Source: three-view drawing plus pictorial views. Frame: mm from the lowest corner of the part. Give positions to 0.01 mm unless a question says otherwise; leave off trailing zeros. Write each loop counter-clockwise with the first axis right and the second up, starting at its lowest first coordinate (ties: lowest second). Pieces come first, ordered by that corner, then holes. Notation, with made-up numbers: (86, -3) -> (135, -3) arc R11 ccw to (135, 14) -> close; hole circle Ø11 at (41, 70.5). An arc over 180 degrees is marked (long way). Use a Markdown table: item, result. Add a question column.
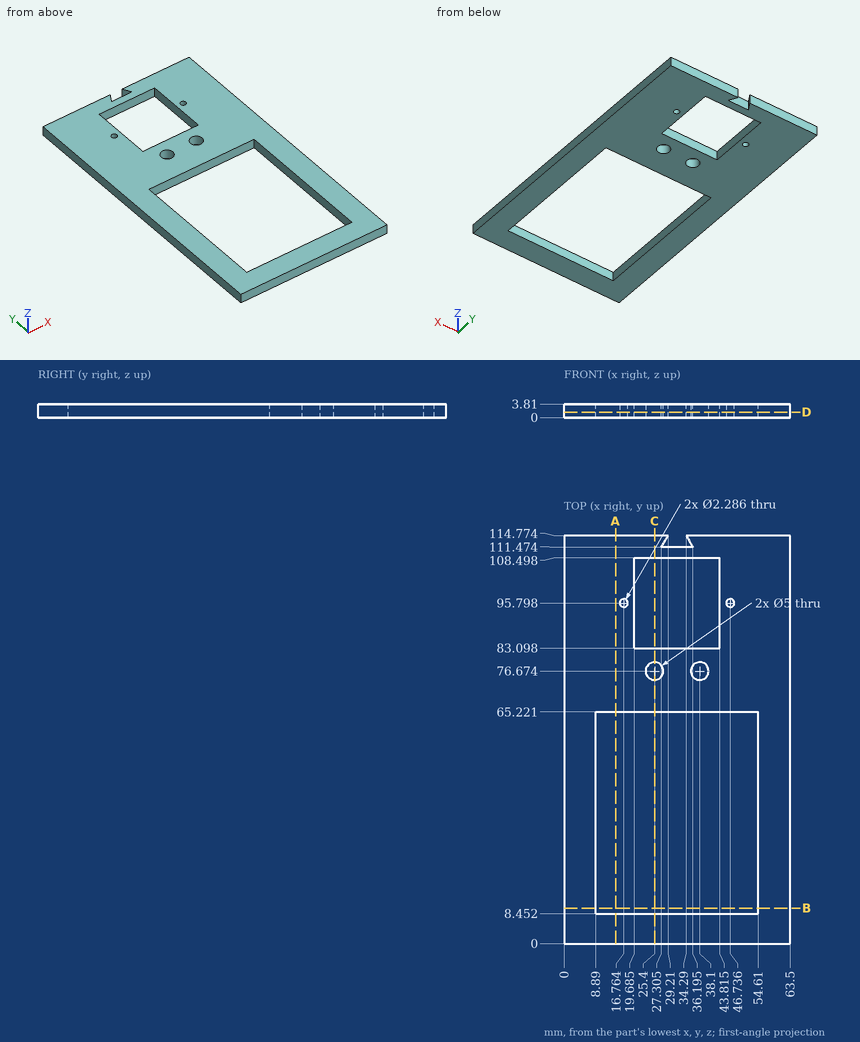
(1) First-contact query: pin 1 Ø1.1 at (x, z) = (30.5, 2) entering from +Y; pin 2 Ø1.4 at (x, y) = (46.74, 95.8) entering from -Z. Flat tips, straight axial feed; report the tip coordinate or a pass-through.
(2) Cut plane C-C on x = 25.4. Return the cut outline in (y, z), then the cut area to 3 significant figures.
(3) Cut plane D-D on z = 1.55. Return the cut outline in (x, y) (1 decimal).
(4) Material intervals for L1, parallel to Y at x = 25.4, z = 1; L2, parallel to Y at x = 22, z = 0.6; L3, parallel to Y at x = 29.5, z = 2.8 (1 decimal), sorted ascending.
(5) Cut plane A-A on x = 14.5. Return the cut outline in (y, z), then the cut area to 3 significant figures.
(6) Cut plane B-B on y = 10. Return the cut outline in (x, z).
Output:
| question | item | result |
|---|---|---|
| 1 | pin 1 | y = 111.47 |
| 1 | pin 2 | through |
| 2 | outline | (0, 0) -> (8.45, 0) -> (8.45, 3.81) -> (0, 3.81) -> close; (65.22, 0) -> (74.17, 0) -> (74.17, 3.81) -> (65.22, 3.81) -> close; (79.17, 0) -> (83.1, 0) -> (83.1, 3.81) -> (79.17, 3.81) -> close; (108.5, 0) -> (114.77, 0) -> (114.77, 3.81) -> (108.5, 3.81) -> close |
| 2 | area | 105 mm^2 |
| 3 | outline | (0, 0) -> (63.5, 0) -> (63.5, 114.8) -> (34.3, 114.8) -> (36.2, 111.5) -> (27.3, 111.5) -> (29.2, 114.8) -> (0, 114.8) -> close; hole (8.9, 8.5) -> (54.6, 8.5) -> (54.6, 65.2) -> (8.9, 65.2) -> close; hole circle Ø2.3 at (16.8, 95.8); hole (19.7, 83.1) -> (43.8, 83.1) -> (43.8, 108.5) -> (19.7, 108.5) -> close; hole circle Ø5 at (25.4, 76.7); hole circle Ø5 at (38.1, 76.7); hole circle Ø2.3 at (46.7, 95.8) |
| 4 | L1 | 0 to 8.45, 65.22 to 74.17, 79.17 to 83.1, 108.5 to 114.77 |
| 4 | L2 | 0 to 8.45, 65.22 to 83.1, 108.5 to 114.77 |
| 4 | L3 | 0 to 8.5, 65.2 to 83.1, 108.5 to 111.5 |
| 5 | outline | (0, 0) -> (8.45, 0) -> (8.45, 3.81) -> (0, 3.81) -> close; (65.22, 0) -> (114.77, 0) -> (114.77, 3.81) -> (65.22, 3.81) -> close |
| 5 | area | 221 mm^2 |
| 6 | outline | (0, 0) -> (8.89, 0) -> (8.89, 3.81) -> (0, 3.81) -> close; (54.61, 0) -> (63.5, 0) -> (63.5, 3.81) -> (54.61, 3.81) -> close |
